The figure shows three views and two pictorial views of one solid part (mm, origin at its lowest corner). Answer the questions. A direction names the side the tool comes from. Give positions to 0.01 mm unless a question says otherwise; leave off trailing zeros. Order: outer loops, then holes, each group sorted by start corner. A loop starts at its lowest first (then second) coordinate and runs counter-clockwise, first axis right, second up. Notation, with made-up numbers: M 60,44.25 L 113,44.25 A17 cw 113,52.25 Z; hole C 88,66 d10. An arc over 180 degrees is marked long. Write item = value, one per line. Start each with the question number.
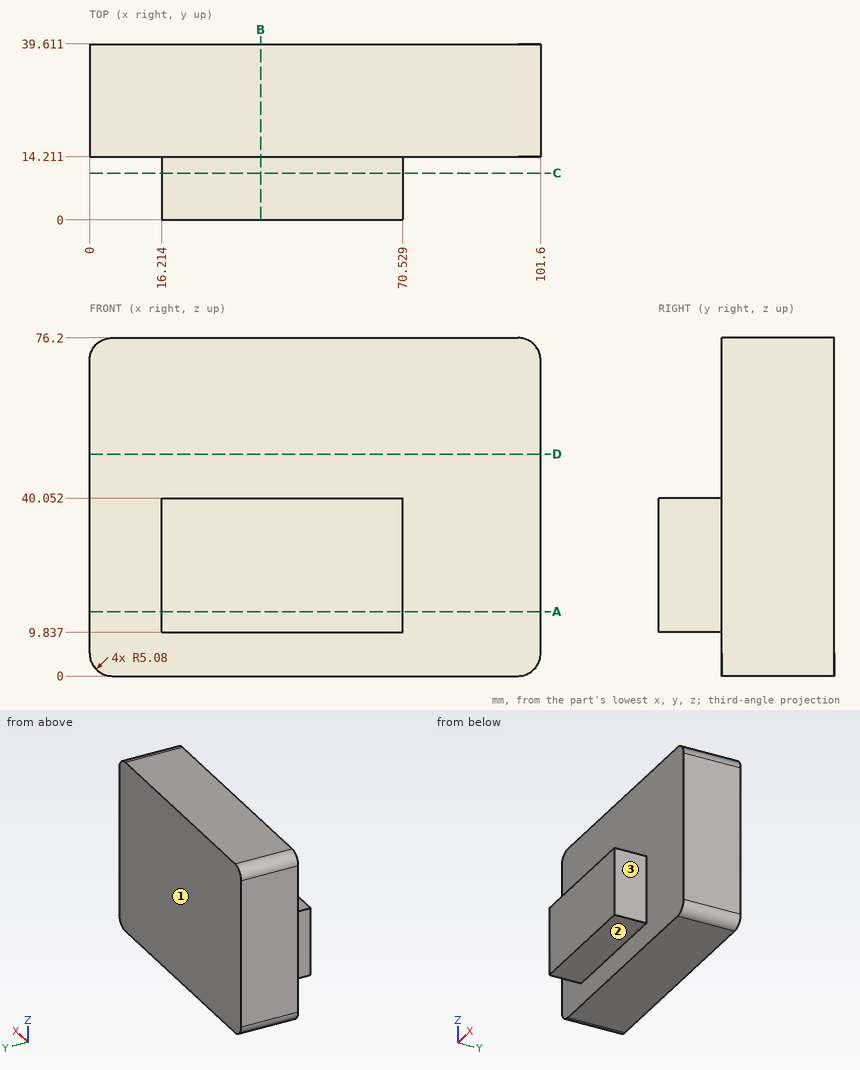
1) Find section D-D on z = 50. Determine the outline of the cut face in (x, y), plus the area to 3 significant figures.
2) Each of these flat-tipped pins is pushed along its axis until it touches: P1, Ø1, axis at y = 13, z = 35, coming from the +X side; P2, Ø11.5, axis at x = 31, y = 4.5, coming from the +Z side; P3, Ø8, axis at y = 8, z = 9.5, coming from the -X side. Where does it stop, or does it pass through?
3) For the marked faces 1, 2 and 3, determine the directions among +Z, -Z, +X, -X, +Y, -Y from which every point of the face is accessible in a straight line to the end or side of a thin tool.
4) Find section A-A on z = 14.5. Determine the outline of the cut face in (x, y), plus the area to 3 significant figures.
5) Find section C-C on y = 10.5. Determine the outline of the cut face in (x, z), plus the area to 3 significant figures.
6) Find section B-B on x = 38.5. Determine the outline of the cut face in (y, z).
7) Find the intervals of material crossed by probe 1 along X at (y, z) = (12, 15); probe 2 along Z at (x, y) = (38.5, 13.5); probe 3 along Y at (x, z) = (53, 65), in increasing order. Write a range as [from, to].
Numbers:
q1.outline = M 0,14.21 L 101.6,14.21 L 101.6,39.61 L 0,39.61 Z
q1.area = 2,580 mm2
q2.P1 = 70.53
q2.P2 = 40.05
q2.P3 = 16.21
q3.face_1 = +Z, -Z, +X, -X, +Y
q3.face_2 = -Z, +X, -X, -Y
q3.face_3 = +Z, -Z, +X, -Y
q4.outline = M 0,14.21 L 16.21,14.21 L 16.21,0 L 70.53,0 L 70.53,14.21 L 101.6,14.21 L 101.6,39.61 L 0,39.61 Z
q4.area = 3,350 mm2
q5.outline = M 16.21,9.84 L 70.53,9.84 L 70.53,40.05 L 16.21,40.05 Z
q5.area = 1,640 mm2
q6.outline = M 0,9.84 L 14.21,9.84 L 14.21,0 L 39.61,0 L 39.61,76.2 L 14.21,76.2 L 14.21,40.05 L 0,40.05 Z
q7.probe_1 = [16.21, 70.53]
q7.probe_2 = [9.84, 40.05]
q7.probe_3 = [14.21, 39.61]
